Build history of the part. All positions in model axes, mm. Face numbers are marked on the shaded views. A direction names the side the tool comes from. Give positions to 0.01 mm unless a question says otherwise; leave off trailing zeros. Order: outer loops, then holes, each group sorted by start corner. A loop starts at its lowest first (then second) coordinate and runs counter-clockwise, first axis right, second up. Notation, with made-up numbers: (30, 22.25) -> (73, 22.25) arc R12 ccw to (73, 36.25) -> close; hole circle Ø10 at (21, -10). An arc over 180 degrees is marked (long way). One line per item, written item: value. Start each with the question number.
(1) Saw through at C-C on z = 125.25. Give the cut face in (x, y), plus the area to 3 significant figures.
(2) Saw through at D-D on y = 4. Give the cut face in (x, z).
(3) Saw through at A-A on z = 115. Give the cut face in (x, y), plus the area to 3 significant figures.
(4) Saw through at B-B on y = 11. Give the cut face in (x, z), plus the area to 3 significant figures.
(5) Probe line 1 (X direction, y = 9, z = 113); line 2 (Y direction, x = 21, z = 124); line 3 (Y direction, x = 8, z = 112.5). List the from-to ranges inside material, lowest first.
(6) Two-plate mould, pull along Y, no slides. Class the marked faces 3, 4, 5 and 6: +Y half, -Y half, draft (parallel to the pull), parting line (faces both ways), or undercut.
(7) Which spindle directions (+Z, -Z, +X, -X, +Y, -Y) get a long thin tool onto all of the face, cutting with end or side? Do the marked faces 1 and 2. Say none if no direction does.
(8) Pin check, flat tips, straight feed: pin 1 (1.5 mm diameter, centred on y = 10, z = 115, fed in from -X); pin 2 (2 mm diameter, centred on y = 11.5, z = 127.5, fed in from +X); pin 3 (3 mm diameter, centred on x = 32, y = 5.5, fed in from -Z); pin 4 (10 mm diameter, centred on x = 10, y = 19, fed in from +Z). Stop position of each tip, or through.
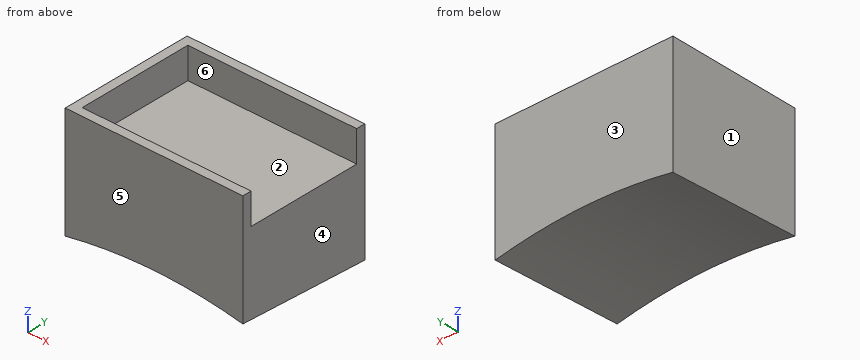
```python
from build123d import *

# Parameters (mm, degrees)
SKETCH1_W           = 40
SKETCH1_H           = 30
BOSS_EXTRUDE1_DEPTH = 130
SKETCH6_W           = 30
SKETCH6_H           = 20
CUT_EXTRUDE1_DEPTH  = 10
SKETCH7_W           = 38
SKETCH7_H           = 26
CUT_EXTRUDE2_DEPTH  = 7


with BuildPart() as part:
    # Sketch1 → Boss-Extrude1 (new body)
    with BuildSketch(Plane.XY):
        with Locations((20, 15)):
            Rectangle(SKETCH1_W, SKETCH1_H)
    extrude(amount=BOSS_EXTRUDE1_DEPTH)

    # Sketch4 → Cut-Revolve1 (revolve, cut)
    with BuildSketch(Plane(origin=(20, 0, 0), x_dir=(0, 0, -1), z_dir=(1, 0, 0))):
        Polygon((0, 60), (0, -170), (-115.503789235, -170), (-103.45, 60), align=None)
    revolve(axis=Axis((20, 60, 0), (0, -1, 0)), mode=Mode.SUBTRACT)

    # Sketch6 → Cut-Extrude1 (cut)
    with BuildSketch(Plane.XY.offset(120)):
        with Locations((20, 15)):
            Rectangle(SKETCH6_W, SKETCH6_H)
    extrude(amount=-CUT_EXTRUDE1_DEPTH, mode=Mode.SUBTRACT)

    # Sketch7 → Cut-Extrude2 (cut)
    with BuildSketch(Plane.XY.offset(130)):
        with Locations((21, 15)):
            Rectangle(SKETCH7_W, SKETCH7_H)
    extrude(amount=-CUT_EXTRUDE2_DEPTH, mode=Mode.SUBTRACT)


solid = part.part
```
Results below:
1. outline: (0, 0) -> (40, 0) -> (40, 2) -> (2, 2) -> (2, 28) -> (40, 28) -> (40, 30) -> (0, 30) -> close
1. area: 212 mm²
2. outline: (0, 104.49) arc R106.38 cw to (40, 104.49) -> (40, 123) -> (2, 123) -> (2, 130) -> (0, 130) -> close
3. outline: (0, 0) -> (40, 0) -> (40, 30) -> (0, 30) -> close; hole (5, 5) -> (35, 5) -> (35, 25) -> (5, 25) -> close
3. area: 600 mm²
4. outline: (0, 104.11) arc R106.02 cw to (40, 104.11) -> (40, 123) -> (2, 123) -> (2, 130) -> (0, 130) -> close; hole (5, 110) -> (35, 110) -> (35, 120) -> (5, 120) -> close
4. area: 419 mm²
5. line 1: x = 0 to 5, 35 to 40
5. line 2: y = 0 to 2, 28 to 30
5. line 3: y = 0 to 5, 25 to 30
6. face 3: +Y half
6. face 4: draft
6. face 5: -Y half
6. face 6: undercut
7. face 1: +Z, -Z, -X, +Y, -Y
7. face 2: +Z, +X
8. pin 1: stops at x = 0
8. pin 2: stops at x = 2
8. pin 3: stops at z = 105.43
8. pin 4: stops at z = 123
